For this review, use the dimensioned drawing (mm, ordinates from the lowest corner) and the shaded views. A direction names the side the tool comes from. Give positions to 0.01 mm unless a question says otherwise; leave off trailing zeros. Loops run counter-clockwise (first coordinate to the right, second up) from the corner with the lowest first, then second, coordinate; pieces in that order, holes last. Notation, with made-up numbers: M -20,-7 L -6,-7 A13 cw -6,2 Z; hole C -16.5,43 d8. An arc over 180 degrees is marked long. Use CSV: the item, a comma, the result in double quotes.
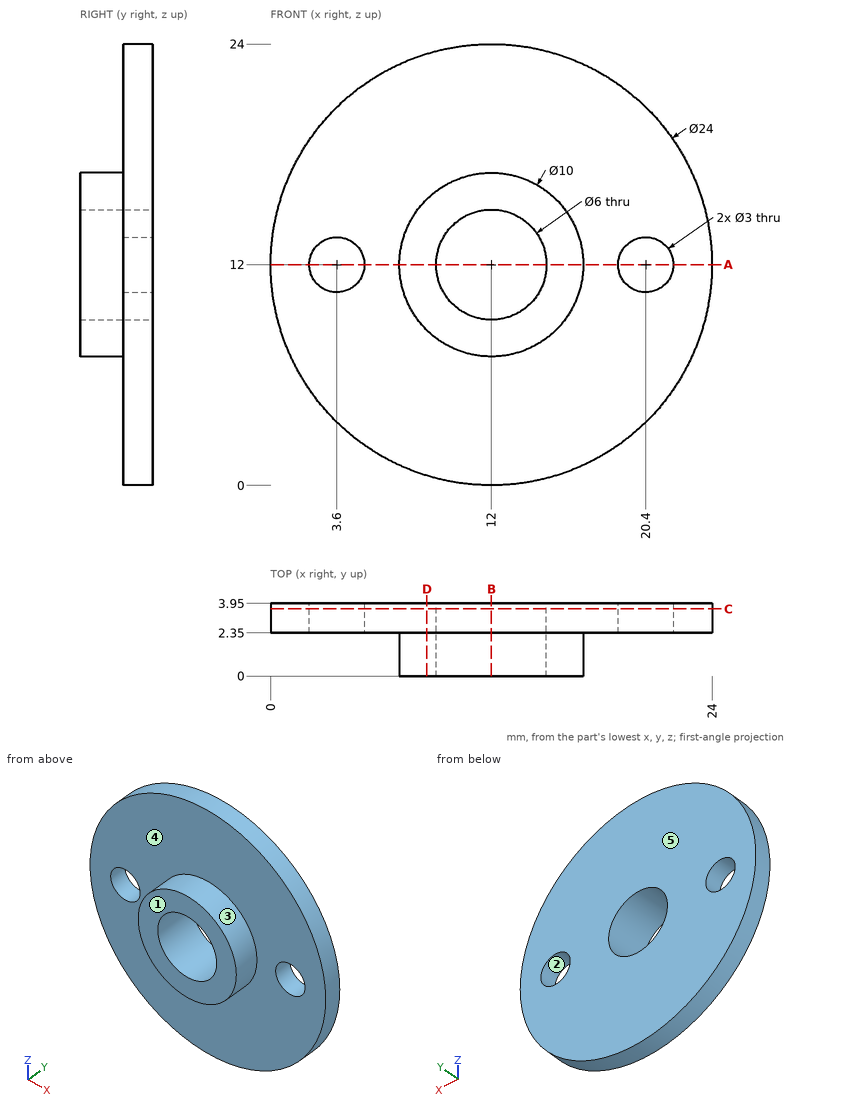
(1) Wall thickness on line 1 along X through (y, z) = (3.05, 12); line 2 along X through (y, z) = (2.2, 12); line 3 along Y through (x, z) = (9.75, 4): over which ranges is each line inside the solid? List them lowest first. Write a range as [from, to].
A:
line 1,"[0, 2.1], [5.1, 9], [15, 18.9], [21.9, 24]"
line 2,"[7, 9], [15, 17]"
line 3,"[2.35, 3.95]"
(2) The part is to be moulded in two halves that separate along X. For the marked faces 1, 2 and 3, say which applies: released by +X, released by -X, zero draft, split by the parting line, or undercut.
A:
face 1,"zero draft"
face 2,"undercut"
face 3,"split by the parting line"
(3) We need section C-C on y = 3.65. State the section outline as (x, z) points.
A:
outline,"C 12,12 d24; hole C 3.6,12 d3; hole C 12,12 d6; hole C 20.4,12 d3"
(4) We need section D-D on x = 8.5. State the section outline as (y, z) points.
A:
outline,"M 0,8.43 L 2.35,8.43 L 2.35,0.52 L 3.95,0.52 L 3.95,23.48 L 2.35,23.48 L 2.35,15.57 L 0,15.57 Z"
(5) We need section A-A on z = 12. State the section outline as (x, y) points, then the cut area to 3 significant figures.
A:
outline,"M 0,2.35 L 2.1,2.35 L 2.1,3.95 L 0,3.95 Z; M 5.1,2.35 L 7,2.35 L 7,0 L 9,0 L 9,3.95 L 5.1,3.95 Z; M 15,0 L 17,0 L 17,2.35 L 18.9,2.35 L 18.9,3.95 L 15,3.95 Z; M 21.9,2.35 L 24,2.35 L 24,3.95 L 21.9,3.95 Z"
area,"28.6 mm²"
(6) Clearance check with flat-ended pins moving along their axes: P1, Ø2.5, axis at x = 3.6, z = 12, coming from the -Y side; P2, Ø1.5, axis at x = 15.5, z = 20.5, coming from the -Y side; P3, Ø1, axis at x = 18.5, y = 2, coming from the -Z side. State where each tip first meets the part, or that it passes through.
A:
P1,"through"
P2,"y = 2.35"
P3,"z = 1.69"
(7) We need section B-B on x = 12. State the section outline as (y, z) points, then the cut area to 3 significant figures.
A:
outline,"M 0,7 L 2.35,7 L 2.35,0 L 3.95,0 L 3.95,9 L 0,9 Z; M 0,15 L 3.95,15 L 3.95,24 L 2.35,24 L 2.35,17 L 0,17 Z"
area,"38.2 mm²"
(8) Machinability: for the marked faces 4 and 5, which of the approach directions +Z, -Z, +X, -X, +Y, -Y give a long, thin tool a straight path to every point of the face, cutting with its end or side? Answer none if there is none.
A:
face 4,"-Y"
face 5,"+Z, -Z, +X, -X, +Y"
